Geometry check sheet. Reference: the model listing, model coordinates, mm. Face numbers are marked on the shaded views. A direction names the side the tool comes from. Round coordinates to 2 decimals unless told otherwise and drop trailing zeros.
(1) Material ranges on line 1 along X through (y, z) = (6.5, 13.5); line 2 along Z through (x, y) = (19, 6); line 3 along Z through (x, y) = (-15, 8.5), recorded low to high.
(2) Release check for a two-part mould opening along Z. For the marked faces 1, 2 and 3 record: +Z half, -Z half, draft (parallel to the pull), parting line (faces both ways), or undercut.
(3) Set-up check for the marked faces 4, 5 and 6: record each of +Z, -Z, +X, -X, +Y, -Y from which the full face is reachable in a straight line by a thin tool's end or side.
(4) Sectioned sample at A-A (z = 0). Give the number of separate pieces and of enclosed holes in the cut face, plus the area to 3 significant figures.
(5) Go/stop test with flat-tipped pins: pin 1 (6.5 mm diameter, centred on x = 0, z = 0, fed in from +Y); pin 2 (11 mm diameter, centred on x = 0, z = 0, fed in from -Y); pin 3 (8 mm diameter, centred on x = 1, y = 9, fed in from +Z); pin 4 (25 mm diameter, centred on x = -12.5, z = 7, fed in from -Y). Record where each tip stops, or that it passes through.
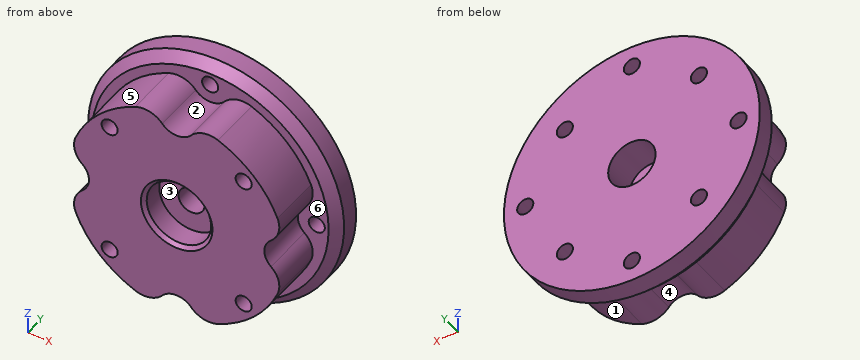
from build123d import *

# Parameters (mm, degrees)
M3_CLEARANCE_HOLE1_D           = 3.4
CUT_EXTRUDE1_DEPTH             = 11.156
FILLET1_R                      = 5
CIRPATTERN1_COUNT              = 4
FILLET1_OF_CIRPATTERN1_R       = 5
CBORE_FOR_M5_SHCS1_D           = 5.5
CBORE_FOR_M5_SHCS1_CBORE_D     = 10
CBORE_FOR_M5_SHCS1_CBORE_DEPTH = 7
CHAMFER1_SIZE                  = 0.75
CHAMFER2_SIZE                  = 2


with BuildPart() as part:
    # Sketch1 → Revolve1 (revolve)
    with BuildSketch(Plane.XY, mode=Mode.PRIVATE) as revolve1_sk:
        Polygon((6.8, 0), (6.8, 4.953), (0, 4.953), (0, 17.156), (27, 17.156), (27, 11.156), (23, 11.156), (23, 0), align=None)
    revolve(revolve1_sk.sketch.rotate(Axis((0, 0, 0), (0, 1, 0)), 90), axis=Axis((0, 0, 0), (0, 1, 0)))

    # M3 Clearance Hole1 (through all)
    with Locations(Plane.XZ):
        with Locations((-14.142135624, -14.142135624), (-22.5, 0)):
            m3_clearance_hole1 = Hole(M3_CLEARANCE_HOLE1_D / 2)

    # Sketch5 → Cut-Extrude1 (cut)
    with BuildSketch(Plane.XZ):
        with BuildLine():
            ThreePointArc((-22.65, -3.997186511), (-18.5, 0), (-22.65, 3.997186511))
            ThreePointArc((-22.65, 3.997186511), (-23, 0), (-22.65, -3.997186511))
        make_face()
    cut_extrude1 = extrude(amount=-CUT_EXTRUDE1_DEPTH, mode=Mode.SUBTRACT)

    # Fillet1
    fillet1_edges = [part.edges().sort_by_distance(p)[0] for p in [
        (-22.65, 5.578, -3.997186511),
        (-22.65, 5.578, 3.997186511),
    ]]
    fillet(fillet1_edges, radius=FILLET1_R)

    # CirPattern1: M3 Clearance Hole1, Cut-Extrude1 ×4 about axis
    cirpattern1_axis = Axis((0, 0, 0), (0, 1, 0))
    add([m3_clearance_hole1.rotate(cirpattern1_axis, i * 360 / CIRPATTERN1_COUNT) for i in range(1, CIRPATTERN1_COUNT)], mode=Mode.SUBTRACT)
    add([cut_extrude1.rotate(cirpattern1_axis, i * 360 / CIRPATTERN1_COUNT) for i in range(1, CIRPATTERN1_COUNT)], mode=Mode.SUBTRACT)

    # Fillet1 of CirPattern1
    fillet1_of_cirpattern1_edges = [part.edges().sort_by_distance(p)[0] for p in [
        (-3.997186511, 5.578, 22.65),
        (3.997186511, 5.578, 22.65),
        (22.65, 5.578, 3.997186511),
        (22.65, 5.578, -3.997186511),
        (3.997186511, 5.578, -22.65),
        (-3.997186511, 5.578, -22.65),
    ]]
    fillet(fillet1_of_cirpattern1_edges, radius=FILLET1_OF_CIRPATTERN1_R)

    # CBORE for M5 SHCS1 (through all)
    with Locations(Plane(origin=(0, 17.156, 0), x_dir=(1, 0, 0), z_dir=(0, 1, 0))):
        with Locations((0, 0)):
            CounterBoreHole(CBORE_FOR_M5_SHCS1_D / 2, CBORE_FOR_M5_SHCS1_CBORE_D / 2, CBORE_FOR_M5_SHCS1_CBORE_DEPTH)

    # Chamfer1
    chamfer1_edges = [part.edges().sort_by_distance(p)[0] for p in [
        (0, 0, 6.8),
    ]]
    chamfer(chamfer1_edges, length=CHAMFER1_SIZE)

    # Chamfer2
    chamfer2_edges = [part.edges().sort_by_distance(p)[0] for p in [
        (0, 11.156, 27),
    ]]
    chamfer(chamfer2_edges, length=CHAMFER2_SIZE)


solid = part.part
Answer below:
1. line 1: x = -18.62 to -15.72, -12.57 to 12.57, 15.72 to 18.62
1. line 2: z = -12.96 to -1.94, 1.94 to 12.96
1. line 3: z = -17.44 to -15.61, -12.67 to 12.67, 15.61 to 17.44
2. face 1: -Z half
2. face 2: +Z half
2. face 3: undercut
3. face 4: -Z, -Y
3. face 5: +Z, -X, -Y
3. face 6: -Y
4. separate pieces: 4
4. enclosed holes: 0
4. area: 525 mm2
5. pin 1: stops at y = 10.16
5. pin 2: stops at y = 4.95
5. pin 3: stops at z = 26.83
5. pin 4: stops at y = 0
